```python
from build123d import *

# Parameters (mm, degrees)
SKETCH1_W           = 2360.422
SKETCH1_H           = 44.45
BOSS_EXTRUDE1_DEPTH = 44.45
SHELL1_T            = -3.175


with BuildPart() as part:
    # Sketch1 → Boss-Extrude1 (new body)
    with BuildSketch(Plane.XY):
        with Locations((1180.211, 22.225)):
            Rectangle(SKETCH1_W, SKETCH1_H)
    extrude(amount=BOSS_EXTRUDE1_DEPTH)

    # Shell1
    shell1_openings = [part.faces().sort_by_distance(p)[0] for p in [
        (2360.422, 22.225, 22.225),
        (0, 22.225, 22.225),
    ]]
    offset(amount=SHELL1_T, openings=shell1_openings, kind=Kind.INTERSECTION)


solid = part.part
```
CAD build for the part. Positions are in the model's coordinates, mm. A direction names the side the tool comes from. Round coordinates to 2 decimals unless told otherwise and drop trailing zeros. Order: outer loops, then holes, each group sorted by start corner. A loop starts at its lowest first (then second) coordinate and runs counter-clockwise, first axis right, second up. Notation, with made-up numbers: (-28, -37.5) - (-8, -37.5) arc R18 cw to (-8, -33.5) - close; hole circle Ø2 at (2.5, -16). An arc over 180 degrees is marked (long way). Use CSV: the item, a comma, the result in double quotes. Start each with the question number.
1) Saw through at A-A (z = 24). List the corners of the cut face in (x, y) (3 decimals).
2) Saw through at C-C (x = 680). List the corners of the cut face in (y, z) (3 decimals).
3) Two-plate mould, pull along Z, no slides. Class faces 1 (the flat face through (1164, 44.45, 22)), 2 (the flat face through (1164, 41.275, 22)), 3 (the flat face through (1164, 23, 44.45)): pulls with the +Z half, pulls with the -Z half, needs draft (parallel to the pull), parting line crosses it, or undercut.
4) Tool access for faces 4 (the flat face through (0, 42, 22)), 5 (the flat face through (1164, 22, 41.275)): list every direction of +Z, -Z, +X, -X, +Y, -Y with a clear straight run to the whole face (end or side of a thin tool).
5) Wall check: L1, parallel to Z at x = 626, y = 35 (3 decimals). Give the ranges that are in metal, low to high. Write a range as [from, to].
Values follow:
1,outline,"(0, 0) - (2360.422, 0) - (2360.422, 3.175) - (0, 3.175) - close; (0, 41.275) - (2360.422, 41.275) - (2360.422, 44.45) - (0, 44.45) - close"
2,outline,"(0, 0) - (44.45, 0) - (44.45, 44.45) - (0, 44.45) - close; hole (3.175, 3.175) - (41.275, 3.175) - (41.275, 41.275) - (3.175, 41.275) - close"
3,face 1,"needs draft"
3,face 2,"undercut"
3,face 3,"pulls with the +Z half"
4,face 4,"+Z, -Z, -X, +Y, -Y"
4,face 5,"+X, -X"
5,L1,"z = [0, 3.175], [41.275, 44.45]"
